```python
from build123d import *

# Parameters (mm, degrees)
REVOLVE1_ANGLE = 180


with BuildPart() as part:
    # Sketch2 → Revolve1 (revolve)
    with BuildSketch(Plane(origin=(0, 0, 0), x_dir=(1, 0, 0), z_dir=(0, 1, 0))):
        Polygon((-28.575, -3.302), (28.575, -3.302), (28.575, -7.302), (18.575, -7.302), (18.575, -6.302), (15.575, -6.302), (15.575, -7.302), (-15.575, -7.302), (-15.575, -6.302), (-18.575, -6.302), (-18.575, -7.302), (-28.575, -7.302), align=None)
    revolve(axis=Axis((-28.575, 0, 0), (1, 0, 0)), revolution_arc=REVOLVE1_ANGLE)


solid = part.part
```
Could you check a few things on this model? Use its own coordinates, in mm. A direction names the side the tool comes from. Coordinates: 2 decimals unless noted, no trailing zeros. Loops run counter-clockwise (first coordinate to the right, second up) from the corner with the lowest first, then second, coordinate; pieces in that order, holes last.
1) Imagine slicing it at C-C (y = -5.75). List the corners of the cut face in (x, z) for me (3 decimals).
Reported:
outline: (-28.575, -4.501) - (-18.575, -4.501) - (-18.575, -2.579) - (-15.575, -2.579) - (-15.575, -4.501) - (15.575, -4.501) - (15.575, -2.579) - (18.575, -2.579) - (18.575, -4.501) - (28.575, -4.501) - (28.575, 4.501) - (18.575, 4.501) - (18.575, 2.579) - (15.575, 2.579) - (15.575, 4.501) - (-15.575, 4.501) - (-15.575, 2.579) - (-18.575, 2.579) - (-18.575, 4.501) - (-28.575, 4.501) - close
2) Imagine slicing it at B-B (z = 0). List the corners of the cut face in (x, y) for me (3 decimals), and give its area (3 significant figures).
Reported:
outline: (-28.575, -7.302) - (-18.575, -7.302) - (-18.575, -6.302) - (-15.575, -6.302) - (-15.575, -7.302) - (15.575, -7.302) - (15.575, -6.302) - (18.575, -6.302) - (18.575, -7.302) - (28.575, -7.302) - (28.575, -3.302) - (-28.575, -3.302) - close
area: 223 mm2
3) Which directions (+Z, -Z, +X, -X, +Y, -Y) give clear straight access to the entire face, cutting with the end or side of a thin tool? Please do faces 4 (the face through (17.1, -6.3, 0.1)), 5 (the face through (0, 0, 5)).
Reported:
face 4: -Y
face 5: +Z, -Z, +X, -X, +Y
4) Thinking about a two-plate mould opening in Z: for faces 1 (the face through (-15.575, -7, 0)), 2 (the face through (-23.6, -7.3, 0.2)), 3 (the face through (0.4, -3.3, 0.1)), which applies, released by +Z, released by -Z, zero draft, split by the parting line, or undercut?
Reported:
face 1: zero draft
face 2: split by the parting line
face 3: undercut
5) Imagine slicing it at D-D (x = -14). List the corners of the cut face in (y, z) for me.
Reported:
outline: (0, -7.3) - (0, -3.3) arc R3.3 cw to (0, 3.3) - (0, 7.3) arc R7.3 ccw to start
6) Will these pins go through, and if not, where does the flat tip stop? pin 1 Ø2 at (y, z) = (-1, -2) entering from +X; pin 2 Ø4 at (x, y) = (4, -3) entering from +Z; pin 3 Ø2 at (x, z) = (-19.5, -4) entering from -Y.
Reported:
pin 1: passes through
pin 2: stops at z = 7.23
pin 3: stops at y = -6.66
7) Please list where these lines run through material, in increasing order: line 1 along X through (y, z) = (-3.75, -5.5) (3 decimals); line 2 along Y through (x, z) = (25.5, 0); line 3 along Z through (x, y) = (-2, -2.5).
Reported:
line 1: x = -28.575 to -18.575, -15.575 to 15.575, 18.575 to 28.575
line 2: y = -7.3 to -3.3
line 3: z = -6.86 to -2.16, 2.16 to 6.86
8) Imagine slicing it at A-A (y = -2). List the corners of the cut face in (x, z) for me (3 decimals), and give its area (3 significant figures).
Reported:
outline: (-28.575, -7.023) - (-18.575, -7.023) - (-18.575, -5.976) - (-15.575, -5.976) - (-15.575, -7.023) - (15.575, -7.023) - (15.575, -5.976) - (18.575, -5.976) - (18.575, -7.023) - (28.575, -7.023) - (28.575, -2.627) - (-28.575, -2.627) - close; (-28.575, 2.627) - (28.575, 2.627) - (28.575, 7.023) - (18.575, 7.023) - (18.575, 5.976) - (15.575, 5.976) - (15.575, 7.023) - (-15.575, 7.023) - (-15.575, 5.976) - (-18.575, 5.976) - (-18.575, 7.023) - (-28.575, 7.023) - close
area: 490 mm2
